Geometry check sheet. Reference: the model listing, model coordinates, mm. Face numbers are marked on the shaded views. A direction names the side the tool comes from. Coordinates: 2 decimals unless noted, no trailing zeros. Order: outer loops, then holes, each group sorted by start corner. A loop starts at its lowest first (then second) coordinate and runs counter-clockwise, first axis right, second up. Notation, with made-up numbers: M 73,-15 L 77,-15 A21 cw 77,-9 Z; hole C 56,81 d5. An arc over 180 degrees is marked long. One line per item, written item: value. Start each with the question number.
1) Draft check along Z on the marked faces 1, 2, 3 and 4. Enter one of: pulls with the +Z half, pulls with the -Z half, needs draft (parallel to the pull), parting line crosses it, or undercut.
2) Sectioned sample at B-B, the plane z = -5. Enter the section's corners in (x, y), then the cut area to 3 significant figures.
3) Sectioned sample at A-A, the plane x = 49.5. Enter the section's corners in (y, z).
4) Sectioned sample at C-C, the plane y = 31. Enter the section's corners in (x, z), then the cut area to 3 significant figures.
5) Access from +Z, -Z, +X, -X, +Y, -Y to the whole of each face (thin tool, end or side, straight path). Record for the marked faces 5 and 6.
6) Thickness scan on L1, parallel to X at y = 66, z = -3.5; L2, parallel to Z at x = 56, y = 54. Record the ranges inside material, lowest first. Write a range as from..to.
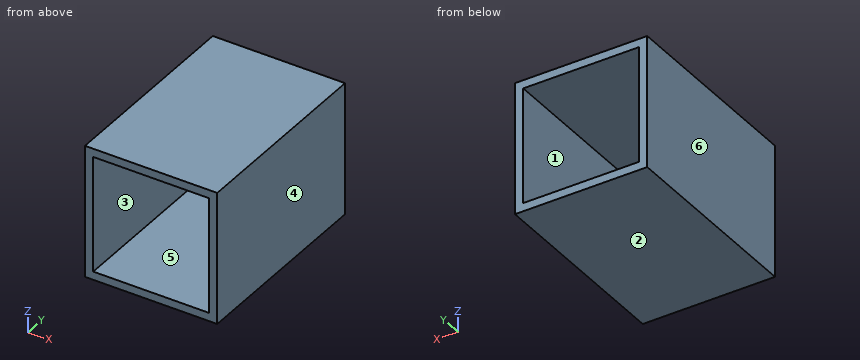
```python
from build123d import *

# Parameters (mm, degrees)
SKETCH1_W           = 50.8
SKETCH1_H           = 50.8
BOSS_EXTRUDE1_DEPTH = 76.2
SHELL1_T            = -3.175


with BuildPart() as part:
    # Sketch1 → Boss-Extrude1 (new body)
    with BuildSketch(Plane(origin=(0, 0, 0), x_dir=(1, 0, 0), z_dir=(0, 1, 0))):
        with Locations((64.927548208, 1.837470194)):
            Rectangle(SKETCH1_W, SKETCH1_H)
    extrude(amount=BOSS_EXTRUDE1_DEPTH)

    # Shell1
    shell1_openings = [part.faces().sort_by_distance(p)[0] for p in [
        (64.927548208, 76.2, -1.837470194),
        (64.927548208, 0, -1.837470194),
    ]]
    offset(amount=SHELL1_T, openings=shell1_openings, kind=Kind.INTERSECTION)


solid = part.part
```
Final values:
1. face 1: undercut
1. face 2: pulls with the -Z half
1. face 3: undercut
1. face 4: needs draft
2. outline: M 39.53,0 L 42.7,0 L 42.7,76.2 L 39.53,76.2 Z; M 87.15,0 L 90.33,0 L 90.33,76.2 L 87.15,76.2 Z
2. area: 484 mm^2
3. outline: M 0,-27.24 L 76.2,-27.24 L 76.2,-24.06 L 0,-24.06 Z; M 0,20.39 L 76.2,20.39 L 76.2,23.56 L 0,23.56 Z
4. outline: M 39.53,-27.24 L 90.33,-27.24 L 90.33,23.56 L 39.53,23.56 Z; hole M 42.7,-24.06 L 87.15,-24.06 L 87.15,20.39 L 42.7,20.39 Z
4. area: 605 mm^2
5. face 5: +Y, -Y
5. face 6: +Z, -Z, -X, +Y, -Y
6. L1: x = 39.53..42.7, 87.15..90.33
6. L2: z = -27.24..-24.06, 20.39..23.56
